Here's how the part is built. I have some questions about the finished solid (model axes, mm). Face numbers are marked on the shaded views. A direction names the side the tool comes from. Give positions to 0.01 mm unless a question says otherwise; leave off trailing zeros. Order: outer loops, then holes, each group sorted by start corner. A loop starts at its lowest first (then second) coordinate and runs counter-clockwise, first axis right, second up.
from build123d import *

# Parameters (mm, degrees)
F1_DEPTH = 6
F2_R     = 8
F5_DEPTH = 45
F3_R     = 4
F6_DEPTH = 6.001
F4_R     = 4
F7_DEPTH = 6.001


with BuildPart() as f1:
    # F0 (on Top) → F1 (new body)
    with BuildSketch(Plane.XY):
        Polygon((19, 57.5), (0, 57.5), (-19, 57.5), (-19, 0), (-19, -57.5), (0, -57.5), (19, -57.5), (19, 0), align=None)
    extrude(amount=F1_DEPTH)

    # F2 (on face) → F5 (join)
    with BuildSketch(Plane.XY.offset(6)):
        with Locations((0, 19.5)):
            Circle(F2_R)
    extrude(amount=F5_DEPTH)

    # F3 (on face) → F6 (cut, through all)
    with BuildSketch(Plane.XY.offset(6)):
        with Locations((0, 39.5)):
            Circle(F3_R)
    extrude(amount=-F6_DEPTH, mode=Mode.SUBTRACT)

    # F4 (on face) → F7 (cut, through all)
    with BuildSketch(Plane.XY.offset(6)):
        with Locations((0, -37.5)):
            Circle(F4_R)
    extrude(amount=-F7_DEPTH, mode=Mode.SUBTRACT)


solid = f1.part
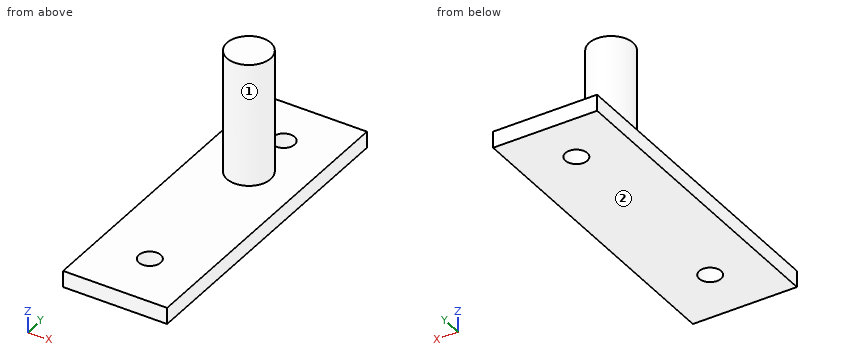
Q1. If we section it at D-D on x = -13: List the corners of the cut face in (y, z) for me, plus the area to 3 significant figures.
Filled sheet:
outline: (-57.5, 0) - (57.5, 0) - (57.5, 6) - (-57.5, 6) - close
area: 690 mm2
Q2. If we section it at C-C on y = -35: List the corners of the cut face in (x, z) for me, plus the area to 3 significant figures.
Filled sheet:
outline: (-19, 0) - (-3.12, 0) - (-3.12, 6) - (-19, 6) - close; (3.12, 0) - (19, 0) - (19, 6) - (3.12, 6) - close
area: 191 mm2
Q3. For the marked faces 1 and 2, which set-ups out of +Z, -Z, +X, -X, +Y, -Y let a thin tool reach every point of the face, with its end or its side?
Filled sheet:
face 1: +Z
face 2: -Z, +X, -X, +Y, -Y
Q4. I'm going to push flat-ended pins straight in: P1, Ø4, axis at x = -0.5, z = 33, coming from the -Y side; P2, Ø7, axis at x = 0, y = -37.5, coming from the -Z side; P3, Ø1.5, axis at y = 14.5, z = 28.5, coming from the -X side; P4, Ø5, axis at x = 2.5, z = 9, coming from the +Y side. Where does each tip first touch, or does it pass through?
Filled sheet:
P1: stops at y = 11.5
P2: passes through
P3: stops at x = -6.78
P4: stops at y = 27.5
Q5. I need wall thicknesses on L1, parallel to Y at x = 0, z = 2.8; L2, parallel to Z at x = 17, y = 34; L3, parallel to X at y = 39, z = 4. Which ranges of each line are inside material? Lowest first, please.
Filled sheet:
L1: y = -57.5 to -41.5, -33.5 to 35.5, 43.5 to 57.5
L2: z = 0 to 6
L3: x = -19 to -3.97, 3.97 to 19
Q6. If we section it at B-B on x = 0: List the corners of the cut face in (y, z) for me, plus the area to 3 significant figures.
Filled sheet:
outline: (-57.5, 0) - (-41.5, 0) - (-41.5, 6) - (-57.5, 6) - close; (-33.5, 0) - (35.5, 0) - (35.5, 6) - (27.5, 6) - (27.5, 51) - (11.5, 51) - (11.5, 6) - (-33.5, 6) - close; (43.5, 0) - (57.5, 0) - (57.5, 6) - (43.5, 6) - close
area: 1,310 mm2
Q7. If we section it at A-A on y = 39.5: List the corners of the cut face in (x, z) for me.
Filled sheet:
outline: (-19, 0) - (-4, 0) - (-4, 6) - (-19, 6) - close; (4, 0) - (19, 0) - (19, 6) - (4, 6) - close
